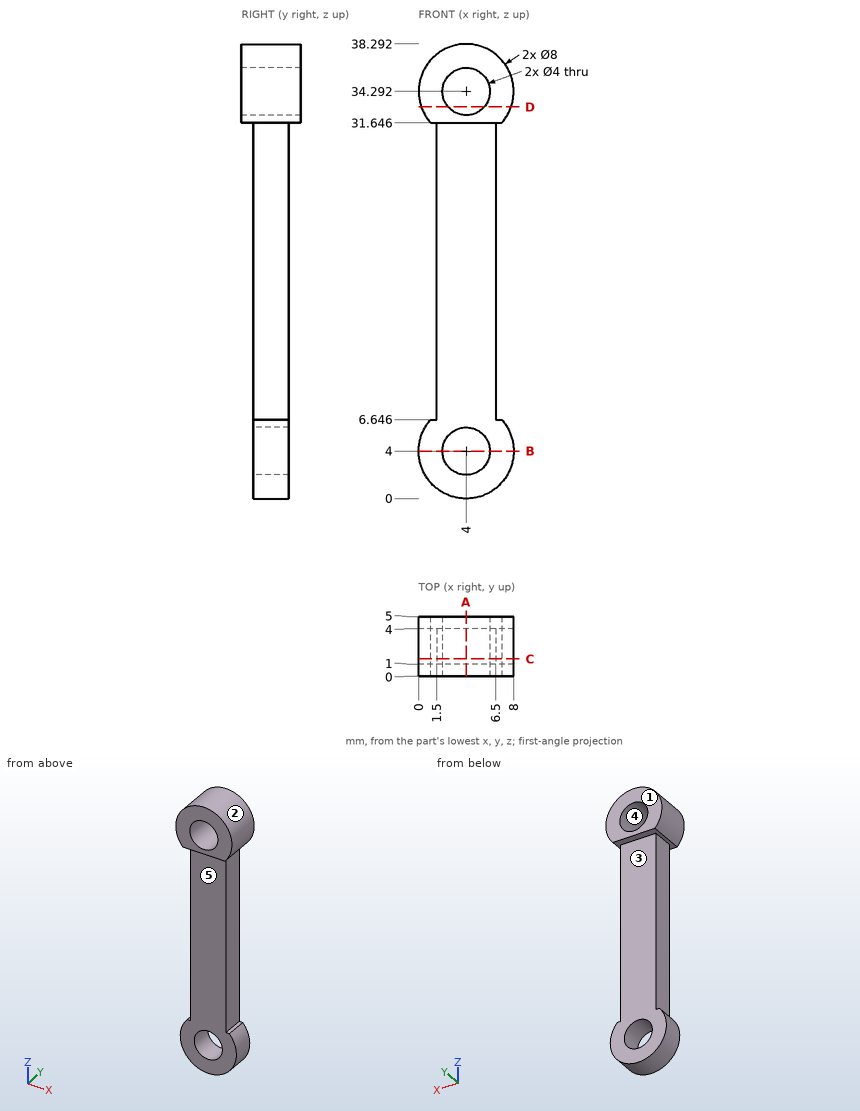
The drawing under review shows one solid part. Ordinate dimensions are in mm from its lowest x, y, z. A direction names the side the tool comes from. Coordinates: 2 decimals unless noted, no trailing zeros. Loops run counter-clockwise (first coordinate to the right, second up) from the corner with the lowest first, then second, coordinate; pieces in that order, holes last. Notation, with made-up numbers: M 67.5,-22.5 L 118.5,-22.5 A30 ccw 118.5,5.5 Z; hole C 29,24.5 d7. An arc over 180 degrees is marked long. Use one line per item in the form item = value.
(1) Consider section C-C (y = 1.45). Write out the cut boundary in (x, z) (1 decimal).
Return value:
outline = M 1,6.6 A4 ccw long 7,6.6 L 6.5,6.6 L 6.5,31.6 L 7,31.6 A4 ccw long 1,31.6 L 1.5,31.6 L 1.5,6.6 Z; hole C 4,4 d4; hole C 4,34.3 d4
(2) Clearance check with flat-ended pins moving along their axes: P1, Ø0.6, axis at x = 1, y = 2, coming from the +Z side; P2, Ø1.5, axis at x = 5.5, y = 3, coming from the -Z side; P3, Ø1, axis at x = 4.5, z = 22, coming from the +Y side; P4, Ø3.5, axis at x = 4, z = 34.29, coming from the -Y side. State where each tip first meets the part, or that it passes through.
Return value:
P1 = 37.24
P2 = 0.07
P3 = 4
P4 = through
(3) For line 1 along Z through (x, y) = (4, 2); line 2 along X through (y, z) = (3.4, 4); line 3 along X through (y, z) = (2.65, 27), list the stretches that pass through material, from the lowest coordinate up. Write a range as from..to.
Return value:
line_1 = 0..2, 6..32.29, 36.29..38.29
line_2 = 0..2, 6..8
line_3 = 1.5..6.5
(4) For the marked faces 3, 4 and 5, list the 3-axis set-ups (+Z, -Z, +X, -X, +Y, -Y) from which the entire face can be reached by the end or side of a thin tool; tool diameter is ignored.
Return value:
face_3 = -Z, +X, -X, +Y
face_4 = +Y, -Y
face_5 = -Z, +X, -X, -Y
(5) Consider section B-B (z = 4). Write out the cut boundary in (x, y), and give its area (3 significant figures).
Return value:
outline = M 0,1 L 2,1 L 2,4 L 0,4 Z; M 6,1 L 8,1 L 8,4 L 6,4 Z
area = 12.0 mm2
(6) Consider section D-D (z = 33). Write out the cut boundary in (x, y) (1 decimal).
Return value:
outline = M 0.2,0 L 2.5,0 L 2.5,5 L 0.2,5 Z; M 5.5,0 L 7.8,0 L 7.8,5 L 5.5,5 Z
(7) Draft analysis for pull direction Z (two halves, no side actions). For the marked faces 1 and 2, state which applies: pulls with the +Z half, pulls with the -Z half, needs draft (parallel to the pull), parting line crosses it, or undercut.
Return value:
face_1 = needs draft
face_2 = undercut
(8) Consider section A-A (x = 4). Write out the cut boundary in (y, z) (1 decimal).
Return value:
outline = M 0,31.6 L 1,31.6 L 1,6 L 4,6 L 4,31.6 L 5,31.6 L 5,32.3 L 0,32.3 Z; M 0,36.3 L 5,36.3 L 5,38.3 L 0,38.3 Z; M 1,0 L 4,0 L 4,2 L 1,2 Z
